from build123d import *

# Parameters (mm, degrees)
SKETCH1_R           = 1.975
SKETCH1_R_2         = 2.1082
BOSS_EXTRUDE1_DEPTH = 4.5


with BuildPart() as part:
    # Sketch1 → Boss-Extrude1 (new body)
    with BuildSketch(Plane(origin=(0, 0, 0), x_dir=(1, 0, 0), z_dir=(0, 1, 0))):
        with BuildLine():
            Line((63, 20.3), (21.8, 20.3))
            ThreePointArc((21.8, 20.3), (20.385786438, 19.714213562), (19.8, 18.3))
            Line((19.8, 18.3), (19.8, 11.37))
            Line((19.8, 11.37), (10.87, 11.37))
            Line((10.87, 11.37), (10.87, 15.95))
            ThreePointArc((10.87, 15.95), (9.595914498, 19.025914498), (6.52, 20.3))
            Line((6.52, 20.3), (-63, 20.3))
            ThreePointArc((-63, 20.3), (-64.414213562, 19.714213562), (-65, 18.3))
            Line((-65, 18.3), (-65, -50.9))
            ThreePointArc((-65, -50.9), (-64.414213562, -52.314213562), (-63, -52.9))
            Line((-63, -52.9), (63, -52.9))
            ThreePointArc((63, -52.9), (64.414213562, -52.314213562), (65, -50.9))
            Line((65, -50.9), (65, 18.3))
            ThreePointArc((65, 18.3), (64.414213562, 19.714213562), (63, 20.3))
        make_face()
        with Locations(Location((-60.5, 15.8, 0), (0, 0, 270))):
            Circle(SKETCH1_R, mode=Mode.SUBTRACT)
        with Locations(Location((60.5, 15.8, 0), (0, 0, 90))):
            Circle(SKETCH1_R, mode=Mode.SUBTRACT)
        with Locations(Location((60.5, -10.3, 0), (0, 0, 270))):
            Circle(SKETCH1_R, mode=Mode.SUBTRACT)
        with Locations(Location((-60.5, -10.3, 0), (0, 0, 90))):
            Circle(SKETCH1_R, mode=Mode.SUBTRACT)
        with Locations(Location((-25.004260819, 16.35, 0), (0, 0, 270))):
            Circle(SKETCH1_R, mode=Mode.SUBTRACT)
        with Locations(Location((-5.328324842, -2.339651524, 0), (0, 0, 270))):
            Circle(SKETCH1_R, mode=Mode.SUBTRACT)
        with Locations(Location((-50.8, -38.838722529, 0), (0, 0, 270))):
            Circle(SKETCH1_R_2, mode=Mode.SUBTRACT)
        with Locations(Location((50.8, -38.838722529, 0), (0, 0, 90))):
            Circle(SKETCH1_R_2, mode=Mode.SUBTRACT)
        with Locations(Location((-43.8023, -2.339651524, 0), (0, 0, 270))):
            Circle(SKETCH1_R_2, mode=Mode.SUBTRACT)
        with Locations(Location((43.8023, -2.339651524, 0), (0, 0, 90))):
            Circle(SKETCH1_R_2, mode=Mode.SUBTRACT)
        with BuildLine():
            Line((-5.328324842, -31.589651524), (-10.508324842, -31.589651524))
            Line((-10.508324842, -31.589651524), (-10.5114167, -11.629651524))
            Line((-10.5114167, -11.629651524), (-5.328324842, -11.629651524))
            ThreePointArc((-5.328324842, -11.629651524), (-1.773195755, -10.922492381), (1.240697155, -8.908673522))
            Line((1.240697155, -8.908673522), (4.903510282, -5.245860395))
            Line((4.903510282, -5.245860395), (19.017361634, -19.359711748))
            Line((19.017361634, -19.359711748), (15.354548508, -23.022524874))
            ThreePointArc((15.354548508, -23.022524874), (5.865165555, -29.36312785), (-5.328324842, -31.589651524))
        make_face(mode=Mode.SUBTRACT)
    extrude(amount=BOSS_EXTRUDE1_DEPTH)


solid = part.part
The model under review builds one solid part; all positions refer to its coordinate system, in mm. A direction names the side the tool comes from. Round coordinates to 2 decimals unless told otherwise and drop trailing zeros. Write each loop counter-clockwise with the first axis right and the second up, starting at its lowest first coordinate (ties: lowest second). Pieces come first, ordered by that corner, then holes. Notation, with made-up numbers: (-24, -5) - (0, -5) arc R18 ccw to (0, 14) - close; hole circle Ø2 at (17.25, 18). An arc over 180 degrees is marked (long way). One line per item, written item: value. Start each with the question number.
1. Consider section C-C on x = 50.8. Write out the cut boundary in (y, z).
2. The part is to be moulded in two halves that separate along Z. For faces 4 (the face through (-1, 2, 52.9)), 5 (the face through (-8, 2, 31.59)), 6 (the face through (-1, 0, 8)), say which applies: released by +Z, released by -Z, zero draft, split by the parting line, or undercut.
3. To check wall thickness, follow L1, parallel to X at y = 1.15, z = -16.35; L2, parallel to X at y = 3.8, z = 10.5; L3, parallel to X at y = 0.45, z = 9.5. State the ranges of each line that lie inside material, in increasing order. Write a range as from..to.
4. Consider section B-B on z = 25.5. Write out the cut boundary in (x, y), and give its area (3 significant figures).
5. Consider section A-A on x = -60.5. Write out the cut boundary in (y, z) (3 decimals), and give its area (3 significant figures).
6. Machinability: for faces 1 (the face through (15, 2, -11.37)), 2 (the face through (-1, 4.5, 8)), 3 (the face through (17.212, 2.218, 21.165)), which of the approach directions +Z, -Z, +X, -X, +Y, -Y give a long, thin tool a straight path to every point of the face, cutting with its end or side? Answer none if there is none.
Checks:
1. outline: (0, -20.3) - (4.5, -20.3) - (4.5, 36.73) - (0, 36.73) - close; (0, 40.95) - (4.5, 40.95) - (4.5, 52.9) - (0, 52.9) - close
2. face 4: released by +Z
2. face 5: undercut
2. face 6: zero draft
3. L1: x = -65..-62.4, -58.6..-26.98, -23.03..10.85, 19.8..58.6, 62.4..65
3. L2: x = -65..-62.46, -58.54..-0.89, 10.16..58.54, 62.46..65
3. L3: x = -65..-62.31, -58.69..0.59, 9.16..58.69, 62.31..65
4. outline: (-65, 0) - (-10.51, 0) - (-10.51, 4.5) - (-65, 4.5) - close; (12.54, 0) - (65, 0) - (65, 4.5) - (12.54, 4.5) - close
4. area: 481 mm^2
5. outline: (0, -20.3) - (4.5, -20.3) - (4.5, -17.775) - (0, -17.775) - close; (0, -13.825) - (4.5, -13.825) - (4.5, 8.325) - (0, 8.325) - close; (0, 12.275) - (4.5, 12.275) - (4.5, 52.9) - (0, 52.9) - close
5. area: 294 mm^2
6. face 1: -Z, +Y, -Y
6. face 2: +Z, -Z, +X, -X, +Y
6. face 3: +Y, -Y
